Autodesk Fusion 360 part; units mm, degrees
sketch "スケッチ1" plane through (0, 0, 0) normal (0, 0, 1) x (1, 0, 0)
  line L0 (-3.5, 163) -> (-86.5, 163)
  line L1 (-86.5, 163) -> (-86.5, -163)
  line L2 (-86.5, -163) -> (-3.5, -163)
  line L3 (86.5, -55) -> (86.5, 155)
  line L4 (82.2546, 155) -> (-86.5, -163) construction
  line L5 (-3.5, 163) -> (-3.5, 155)
  line L6 (-3.5, 155) -> (86.5, 155)
  line L7 (-86.5, -163) -> (-3.5, -163) construction
  line L8 (86.5, -75) -> (-3.5, -163)
  line L9 (86.5, -75) -> (-3.5, -75)
  line L10 (-3.5, -75) -> (-3.5, -55)
  line L11 (-3.5, -55) -> (86.5, -55)
  line L12 (-86.5, 163) -> (29.1871, -55) construction
  line L13 (39.8006, -75) -> (55.7541, -105.0627) construction
  dimension "d2" = 326
  dimension "d5" = 83
  dimension "d7" = 90
  dimension "d8" = 20
extrude "押し出し1" add sketch "スケッチ1" along normal blind 6
chamfer "面取り1" distance 30 angle 45 2 edges at (-86.5, -163, 3) (-86.5, 163, 3)
sketch "スケッチ2" plane through (0, 0, 6) normal (0, 0, 1) x (-1, 0, 0)
  line L0 (56.5, -163) -> (86.5, -133)
  line L1 (86.5, -133) -> (86.5, 133)
  line L2 (86.5, 133) -> (56.5, 163)
  line L3 (56.5, 163) -> (3.5, 163)
  line L4 (3.5, 163) -> (-86.5, 75)
  line L5 (-86.5, 75) -> (3.5, 75)
  line L6 (3.5, 75) -> (3.5, 55)
  line L7 (3.5, 55) -> (-86.5, 55)
  line L8 (-86.5, 55) -> (-86.5, -155)
  line L9 (-86.5, -155) -> (3.5, -155)
  line L10 (3.5, -155) -> (3.5, -163)
  line L11 (3.5, -163) -> (56.5, -163)
  line L12 (-86.5, -155) -> (-46.5, -155) construction
  line L13 (-46.5, -155) -> (-46.5, -110) construction
  line L14 (-46.5, -110) -> (-86.5, -110) construction
  line L15 (-86.5, -110) -> (-86.5, -155) construction
  line L16 (-46.5, -110) -> (-46.5, -50) construction
  line L17 (-46.5, -50) -> (-46.5, 10) construction
  point P0 (-46.5, -110)
  point P1 (-46.5, -50)
  dimension "d12" = 40
  dimension "d13" = 45
  dimension "d14" = 60
  dimension "d15" = 60
hole "穴1" at (46.5, 110, 6) at (46.5, 50, 6) at (46.5, -10, 6) direction (0, 0, -1) diameter 18 end through all
equation "d5 = 30 mm + 53 mm"
Here's how the part is built. I have some questions about the finished solid (model axes, mm). A direction names the side the tool comes from. Coordinates: 2 decimals unless noted, no trailing zeros. Loops run counter-clockwise (first coordinate to the right, second up) from the corner with the lowest first, then second, coordinate; pieces in that order, holes last. Notation, with made-up numbers: (-14, -4) - (25, -4) arc R24 ccw to (25, 8) - close; hole circle Ø11 at (1, 2). An arc over 180 degrees is marked (long way). Return JSON: item names as keys, results as strings. Group by question number.
Item 1: On a 3-axis mill with a long thin cutter (end or side, diameter ignored), from which of +Z, -Z, +X, -X, +Y, -Y can I reach the whole of each face in a straight line? I mean faces 5 (the face through (-1, 2, 0)), 6 (the face through (41, 155, 3)), 7 (the face through (-3.5, -65, 3)). Say none if no direction works.
Item 2: If we section it at A-A on y = -10: Write out the boundary of the cut face in (x, z), and give its area (3 significant figures).
Item 3: If we section it at C-C on x = 25: Write out the boundary of the cut face in (y, z), and give its area (3 significant figures).
Item 4: If we section it at D-D on x = 52: Write out the boundary of the cut face in (y, z).
Item 5: I need wall thicknesses on line 1 (Y direction, x = 46.5, z = 2.2); line 2 (X direction, y = 50, z = 4.7); line 3 (X direction, y = -62.5, z = 4.7). Which ranges of each line are inside material? Lowest first, please. Write a range as from..to.
Item 6: If we section it at B-B on z = 2: Write out the boundary of the cut face in (x, y), and give its area (3 significant figures).
Item 7: Will these pins go through, and if not, where does the flat tip stop? P1, Ø3, axis at x = 20.5, z = 3.5, coming from the -Y side; P2, Ø3, axis at y = 159.5, z = 3.5, coming from the +X side; P3, Ø2, axis at x = 55.5, z = 5, coming from the +Y side; P4, Ø16, axis at x = 46.5, y = 110, coming from the +Z side.
Item 8: We'd pull the mould along Y, two halves only. Please class faces 1 (the face through (-71.3, 148.2, 3)), 2 (the face through (-3.5, 159, 3)), 3 (the face through (41, -55, 3)), 4 (the face through (-30, -163, 3)): +Y half, -Y half, draft (parallel to the pull), parting line (faces both ways), or undercut.
Calculated:
{
 "1": {"face 5": "-Z, +X, -X, +Y, -Y", "face 6": "+Z, -Z, +X, +Y", "face 7": "+Z, -Z, +X"},
 "2": {"outline": "(-86.5, 0) - (37.5, 0) - (37.5, 6) - (-86.5, 6) - close; (55.5, 0) - (86.5, 0) - (86.5, 6) - (55.5, 6) - close", "area": "930 mm^2"},
 "3": {"outline": "(-135.13, 0) - (-75, 0) - (-75, 6) - (-135.13, 6) - close; (-55, 0) - (155, 0) - (155, 6) - (-55, 6) - close", "area": "1,620 mm^2"},
 "4": {"outline": "(-108.73, 0) - (-75, 0) - (-75, 6) - (-108.73, 6) - close; (-55, 0) - (-17.12, 0) - (-17.12, 6) - (-55, 6) - close; (-2.88, 0) - (42.88, 0) - (42.88, 6) - (-2.88, 6) - close; (57.12, 0) - (102.88, 0) - (102.88, 6) - (57.12, 6) - close; (117.12, 0) - (155, 0) - (155, 6) - (117.12, 6) - close"},
 "5": {"line 1": "y = -114.11..-75, -55..-19, -1..41, 59..101, 119..155", "line 2": "x = -86.5..37.5, 55.5..86.5", "line 3": "x = -86.5..-3.5"},
 "6": {"outline": "(-86.5, -133) - (-56.5, -163) - (-3.5, -163) - (86.5, -75) - (-3.5, -75) - (-3.5, -55) - (86.5, -55) - (86.5, 155) - (-3.5, 155) - (-3.5, 163) - (-56.5, 163) - (-86.5, 133) - close; hole circle Ø18 at (46.5, -10); hole circle Ø18 at (46.5, 50); hole circle Ø18 at (46.5, 110)", "area": "48,300 mm^2"},
 "7": {"P1": "stops at y = -141", "P2": "stops at x = -3.5", "P3": "stops at y = 155", "P4": "passes through"},
 "8": {"face 1": "+Y half", "face 2": "draft", "face 3": "undercut", "face 4": "-Y half"}
}
